Design review of the part built by this model. Coordinates are the model's own, in mm. Round coordinates to 2 decimals unless told otherwise and drop trailing zeros. Write each loop counter-clockwise with the first axis right and the second up, starting at its lowest first coordinate (ties: lowest second). Pieces come first, ordered by that corner, then holes. Notation, with made-up numbers: M -23,-38 L -6,-38 A29 ccw -6,-6 Z; hole C -37,1.25 d6. An arc over 180 degrees is marked long. Use CSV: the item, a comma, the result in double quotes.
Autodesk Inventor part; units mm, degrees
ref_plane "YZ Plane" through (0, 0, 0) normal (1, 0, 0) x (0, 1, 0)
ref_plane "XZ Plane" through (0, 0, 0) normal (0, 1, 0) x (-1, 0, 0)
sketch "Sketch2" plane through (0, 0, 0) normal (0, 1, 0) x (-1, 0, 0)
  circle A0 centre (0, 0) radius 25
  circle A1 centre (0, 0) radius 23
  dimension "d0" = 50
  dimension "d1" = 46
extrude "Extrusion1" add sketch "Sketch2" along normal blind 600
ref_plane "Work Plane1" through (0, 0, -25) normal (0, 0, 1) x (1, 0, 0)
sketch "Sketch3" plane through (0, 0, -25) normal (0, 0, 1) x (1, 0, 0)
  line L0 (-25, 0) -> (-25, 600)
  line L1 (25, 0) -> (-25, 0)
  line L2 (1.6, 20) -> (-1.6, 20)
  line L3 (-1.6, 20) -> (-1.6, 75)
  line L4 (-1.6, 75) -> (1.6, 75)
  line L5 (1.6, 75) -> (1.6, 20)
  point P0 (0, 0)
  point P1 (0, 75)
  dimension "d4" = 600
  dimension "d5" = 50
  dimension "d6" = 3.2
  dimension "d7" = 55
  dimension "d8" = 20
  dimension "d9" = 25
extrude "Extrusion2" cut sketch "Sketch3" along normal mid plane 10
sketch "Sketch4" plane through (0, 0, 0) normal (0, 1, 0) x (-1, 0, 0)
  circle A0 centre (0, 0) radius 25
  line L0 (0, -25) -> (-21.65, 12.4989) construction
  line L1 (-21.65, 12.4989) -> (21.65, 12.4989) construction
  line L2 (21.65, 12.4989) -> (0, -25) construction
  line L3 (-17.6606, 19.4109) -> (-26.5815, 3.9594) construction
  line L4 (20.7261, 14.1013) -> (22.5717, 10.9047) construction
  dimension "d12" = 43.3
  dimension "d13" = 43.3
  dimension "d14" = 43.3
pattern_circular "Circular Pattern1" count 3 over 360 about axis through (0, 0, 0) along (0, 1, 0) of "Extrusion2"
ref_plane "Work Plane14" through (0, 230, 0) normal (0, -1, 0) x (1, 0, 0)
split_face "Split7"
equation "\"d12\" = d14"
equation "\"d14\" = d13"
1) The part is to be moulded in two halves that separate along Z. For faces 1 (the face through (-22.1, 600, -7.3)), 2 (the face through (2.994, 295.8, -22.804)), 3 (the face through (-23.846, 295.8, -7.509)), say which applies: released by +Z, released by -Z, zero draft, split by the parting line, or undercut.
Answers:
face 1,"zero draft"
face 2,"undercut"
face 3,"split by the parting line"
2) Add section C-C on y = 350. Write out the cut boundary in (x, z).
Answers:
outline,"C 0,0 d50; hole C 0,0 d46"
3) Wall thickness on line 1 along Z through (x, y) = (0.5, 98) (3 decimals); line 2 along X through (y, z) = (431, 10); line 3 along Y through (x, z) = (21.5, 12): over which ranges is each line inside the solid? List them lowest first. Write a range as [from, to].
Answers:
line 1,"[-24.995, -22.995], [22.995, 24.995]"
line 2,"[-22.91, -20.71], [20.71, 22.91]"
line 3,"[0, 20], [75, 600]"
4) Add section B-B on x = 13.5. Write out the cut boundary in (y, z).
Answers:
outline,"M 0,-21.04 L 600,-21.04 L 600,-18.62 L 0,-18.62 Z; M 0,18.62 L 600,18.62 L 600,21.04 L 0,21.04 Z"
5) For pin 1 Ø5 at (x, z) = (15.5, 16) entering from -Y; pin 2 Ø6 at (y, z) = (513.5, -10) entering from -X; pin 3 Ø1.6 at (y, z) = (40.5, -24) entering from +X; pin 4 Ø4 at (x, y) = (-19.5, 471.5) entering from -Z, all flat-tipped, find the tip position at first contact; note any pin that passes through.
Answers:
pin 1,"y = 0"
pin 2,"x = -24"
pin 3,"x = 9.31"
pin 4,"z = -17.85"
6) Add section A-A on z = 0. Write out the cut boundary in (x, y), then the cut area to 3 significant figures.
Answers:
outline,"M -25,0 L -23,0 L -23,600 L -25,600 Z; M 23,0 L 25,0 L 25,600 L 23,600 Z"
area,"2,400 mm²"
